Can you work these out from the drawing? Everything is in mm from the part's minimum corner. Round coordinates to 2 decimals unless told otherwise and drop trailing zeros. Loops run counter-clockwise (first coordinate to the right, second up) from the corner with the lowest first, then second, coordinate; pieces in that order, holes last. Notation, with made-up numbers: (87.25, -36) - (115.25, -36) arc R34 ccw to (115.25, -5) - close; hole circle Ø6 at (19, 5). An arc over 180 degrees is marked (long way). Return JSON: item names as keys, results as strings. Group by question number.
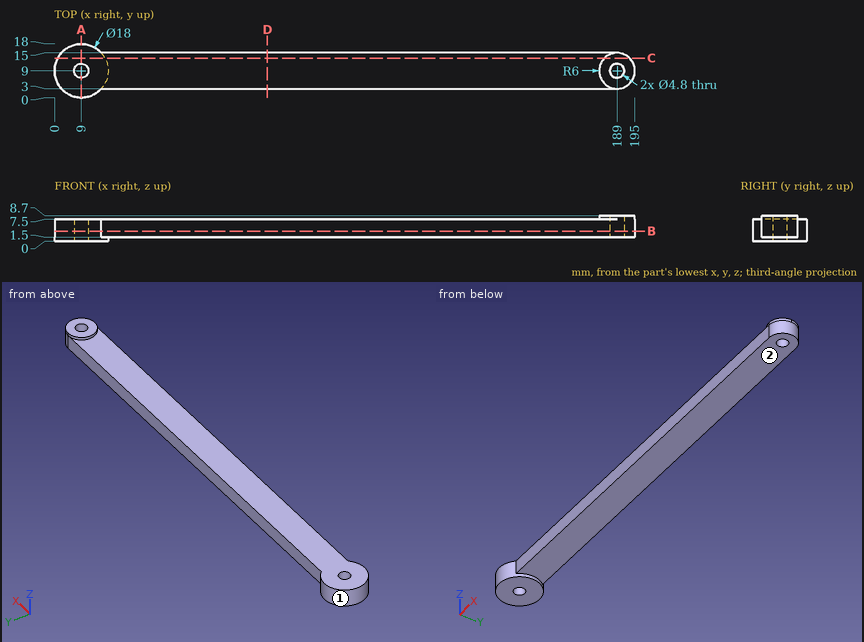
Q1. Imagine slicing it at D-D, the plane x = 71.5. List the corners of the cut face in (y, z) for me, and give its area (3 significant figures).
Q2. Imagine slicing it at C-C, the plane y = 13.25. List the corners of the cut face in (x, z) for me, and give its area (3 significant figures).
Q3. Will these pins go through, and if not, where does the flat tip stop? pin 1 Ø4 at (x, z) = (93, 5.5) entering from -Y; pin 2 Ø6 at (x, y) = (9, 9) entering from -Z; pin 3 Ø1.5 at (y, z) = (14, 6) entering from -X; pin 4 Ø1.5 at (x, y) = (41, 14) entering from +Z.
Q4. Please list where these lines run through material, in increasing order: line 1 (Y direction, x = 9, z = 2.5); line 2 (Z direction, x = 50, y = 6.5); line 3 (X direction, y = 10, z = 4).
Q5. Imagine slicing it at A-A, the plane x = 9. List the corners of the cut face in (y, z) for me, and give its area (3 significant figures).
Q6. Imagine slicing it at B-B, the plane z = 3.5. List the corners of the cut face in (x, y) for me.
Q7. If we mould it in two halves opening along X, with no side actions, what happens to the marked faces 1 and 2? For each: +X half, -X half, draft (parallel to the pull), parting line (faces both ways), or undercut.
Output values:
{
 "1": {"outline": "(3, 1.5) - (15, 1.5) - (15, 7.5) - (3, 7.5) - close", "area": "72.0 mm^2"},
 "2": {"outline": "(1.07, 0) - (16.93, 0) - (16.93, 1.5) - (193.24, 1.5) - (193.24, 8.7) - (184.76, 8.7) - (184.76, 7.5) - (1.07, 7.5) - close", "area": "1,190 mm^2"},
 "3": {"pin 1": "stops at y = 3", "pin 2": "stops at z = 0", "pin 3": "stops at x = 1.07", "pin 4": "stops at z = 7.5"},
 "4": {"line 1": "y = 0 to 6.6, 11.4 to 18", "line 2": "z = 1.5 to 7.5", "line 3": "x = 0.06 to 6.82, 11.18 to 186.82, 191.18 to 194.92"},
 "5": {"outline": "(0, 0) - (6.6, 0) - (6.6, 7.5) - (0, 7.5) - close; (11.4, 0) - (18, 0) - (18, 7.5) - (11.4, 7.5) - close", "area": "99.0 mm^2"},
 "6": {"outline": "(15.71, 3) - (189, 3) arc R6 ccw to (189, 15) - (15.71, 15) arc R9 ccw (long way) to start; hole circle Ø4.8 at (9, 9); hole circle Ø4.8 at (189, 9)"},
 "7": {"face 1": "parting line", "face 2": "draft"}
}
